Source: CAD feature listing. Evaluate the final solid. Frame: model axes, mm. Face numbers are marked on the shaded views. A direction names the side the tool comes from. Round coordinates to 2 decimals unless told otherwise and drop trailing zeros. Write each loop counter-clockwise with the first axis right and the second up, starting at its lowest first coordinate (ties: lowest second). Pieces come first, ordered by that corner, then holes.
from build123d import *

# Parameters (mm, degrees)
ESQUISSE1_W                     = 500
ESQUISSE1_H                     = 240
EXTRUSION1_DEPTH                = 2
ESQUISSE2_R                     = 36
EXTRUSION2_DEPTH                = 2
ESQUISSE3_R                     = 5
ENL_V_MAT_EXTRU_1_DEPTH         = 2
EXTRUSION3_DEPTH                = 500
CONG_1_R                        = 2
ESQUISSE5_R                     = 3.25
ENL_V_MAT_EXTRU_2_DEPTH         = 2
ENL_V_MAT_EXTRU_3_DEPTH         = 2
R_P_TITION_LIN_AIRE1_COUNT      = 2
R_P_TITION_LIN_AIRE1_PITCH      = 101
R_P_TITION_LIN_AIRE1_COUNT_DIR2 = 2
R_P_TITION_LIN_AIRE1_PITCH_DIR2 = 55
ENL_V_MAT_EXTRU_4_DEPTH         = 2
R_P_TITION_LIN_AIRE2_COUNT      = 2
R_P_TITION_LIN_AIRE2_PITCH      = 55
R_P_TITION_LIN_AIRE2_COUNT_DIR2 = 2
R_P_TITION_LIN_AIRE2_PITCH_DIR2 = 101
ESQUISSE8_R                     = 2.75
ENL_V_MAT_EXTRU_5_DEPTH         = 2
ESQUISSE9_R                     = 2.75
ENL_V_MAT_EXTRU_6_DEPTH         = 2
ESQUISSE10_R                    = 1.6
ENL_V_MAT_EXTRU_7_DEPTH         = 394.248331319
ESQUISSE11_R                    = 2.25
ENL_V_MAT_EXTRU_8_DEPTH         = 10


with BuildPart() as part:
    # Esquisse1 → Extrusion1 (new body)
    with BuildSketch(Plane.XY):
        Rectangle(ESQUISSE1_W, ESQUISSE1_H)
    extrude(amount=EXTRUSION1_DEPTH)

    # Esquisse2 → Extrusion2 (add)
    with BuildSketch(Plane.ZY.offset(250)):
        with BuildLine():
            Line((122, -152.166849215), (122, -175.698605572))
            ThreePointArc((122, -175.698605572), (55.48059391, -159.938789336), (0, -120))
            Line((0, -120), (0, 120))
            ThreePointArc((0, 120), (55.48059391, 159.938789336), (122, 175.698605572))
            Line((122, 175.698605572), (122, 152.166849215))
            ThreePointArc((122, 152.166849215), (247.5, 0), (122, -152.166849215))
        make_face()
        with Locations(Location((92.5, 0, 0), (0, 0, 270))):
            Circle(ESQUISSE2_R, mode=Mode.SUBTRACT)
    extrusion2 = extrude(amount=EXTRUSION2_DEPTH)

    # Esquisse3 → Enlèv. mat.-Extru.1 (cut)
    with BuildSketch(Plane.ZY.offset(252)):
        with Locations(Location((110, 140, 0), (0, 0, 270))):
            Circle(ESQUISSE3_R)
        with Locations(Location((110, -140, 0), (0, 0, 90))):
            Circle(ESQUISSE3_R)
    enl_v_mat_extru_1 = extrude(amount=-ENL_V_MAT_EXTRU_1_DEPTH, mode=Mode.SUBTRACT)

    # Symétrie1: Extrusion2, Enlèv. mat.-Extru.1 across plane
    add(extrusion2.mirror(Plane(origin=(0, 0, 0), x_dir=(0, 0, 1), z_dir=(1, 0, 0))))
    add(enl_v_mat_extru_1.mirror(Plane(origin=(0, 0, 0), x_dir=(0, 0, 1), z_dir=(1, 0, 0))), mode=Mode.SUBTRACT)

    # Esquisse4 → Extrusion3 (add)
    with BuildSketch(Plane(origin=(-250, 0, 0), x_dir=(0, 0, -1), z_dir=(1, 0, 0))):
        Polygon((-2, -120), (-67.268218737, -139.080346508), (-66.707032075, -141), (0, -121.499034429), (0, -120), align=None)
    extrusion3 = extrude(amount=EXTRUSION3_DEPTH)

    # Symétrie2: Extrusion3 across plane
    add(extrusion3.mirror(Plane.ZX))

    # Congé1
    cong_1_edges = [part.edges().sort_by_distance(p)[0] for p in [
        (-252, 0, 0),
        (252, 0, 0),
        (0, -121.499034429, 0),
        (0, 121.499034429, 0),
    ]]
    fillet(cong_1_edges, radius=CONG_1_R)

    # Esquisse5 → Enlèv. mat.-Extru.2 (cut)
    with BuildSketch(Plane.XY.offset(2)):
        with Locations((-48, 28)):
            Circle(ESQUISSE5_R)
        with Locations(Location((48, 28, 0), (0, 0, 180))):
            Circle(ESQUISSE5_R)
        with Locations((48, -28)):
            Circle(ESQUISSE5_R)
        with Locations(Location((-48, -28, 0), (0, 0, 180))):
            Circle(ESQUISSE5_R)
    extrude(amount=-ENL_V_MAT_EXTRU_2_DEPTH, mode=Mode.SUBTRACT)

    # Esquisse6 → Enlèv. mat.-Extru.3 (cut)
    with BuildSketch(Plane.XY.offset(2)):
        with BuildLine():
            Line((189, 85), (196, 85))
            ThreePointArc((196, 85), (200, 81), (196, 77))
            Line((196, 77), (189, 77))
            ThreePointArc((189, 77), (185, 81), (189, 85))
        make_face()
    enl_v_mat_extru_3 = extrude(amount=-ENL_V_MAT_EXTRU_3_DEPTH, mode=Mode.SUBTRACT)

    # Répétition linéaire1: Enl_v. mat.-Extru.3 2 × 2
    with Locations(*[(-j * R_P_TITION_LIN_AIRE1_PITCH_DIR2, -i * R_P_TITION_LIN_AIRE1_PITCH, 0) for i in range(R_P_TITION_LIN_AIRE1_COUNT) for j in range(R_P_TITION_LIN_AIRE1_COUNT_DIR2) if (i, j) != (0, 0)]):
        add(enl_v_mat_extru_3, mode=Mode.SUBTRACT)

    # Esquisse7 → Enlèv. mat.-Extru.4 (cut)
    with BuildSketch(Plane.XY.offset(2)):
        with BuildLine():
            Line((-196, -77), (-189, -77))
            ThreePointArc((-189, -77), (-185, -81), (-189, -85))
            Line((-189, -85), (-196, -85))
            ThreePointArc((-196, -85), (-200, -81), (-196, -77))
        make_face()
    enl_v_mat_extru_4 = extrude(amount=-ENL_V_MAT_EXTRU_4_DEPTH, mode=Mode.SUBTRACT)

    # Répétition linéaire2: Enl_v. mat.-Extru.4 2 × 2
    with Locations(*[(i * R_P_TITION_LIN_AIRE2_PITCH, j * R_P_TITION_LIN_AIRE2_PITCH_DIR2, 0) for i in range(R_P_TITION_LIN_AIRE2_COUNT) for j in range(R_P_TITION_LIN_AIRE2_COUNT_DIR2) if (i, j) != (0, 0)]):
        add(enl_v_mat_extru_4, mode=Mode.SUBTRACT)

    # Esquisse8 → Enlèv. mat.-Extru.5 (cut)
    with BuildSketch(Plane.XY.offset(2)):
        with Locations((-241, 87.5)):
            Circle(ESQUISSE8_R)
        with Locations((-71, 87.5)):
            Circle(ESQUISSE8_R)
    extrude(amount=-ENL_V_MAT_EXTRU_5_DEPTH, mode=Mode.SUBTRACT)

    # Esquisse9 → Enlèv. mat.-Extru.6 (cut)
    with BuildSketch(Plane.XY.offset(2)):
        with Locations((71, -87.5)):
            Circle(ESQUISSE9_R)
        with Locations((241, -87.5)):
            Circle(ESQUISSE9_R)
    extrude(amount=-ENL_V_MAT_EXTRU_6_DEPTH, mode=Mode.SUBTRACT)

    # Esquisse10 → Enlèv. mat.-Extru.7 (cut, through all)
    with BuildSketch(Plane.XY.offset(2)):
        with Locations((-169, 48)):
            Circle(ESQUISSE10_R)
        with Locations((-161, 48)):
            Circle(ESQUISSE10_R)
        with Locations((161, -48)):
            Circle(ESQUISSE10_R)
        with Locations((169, -48)):
            Circle(ESQUISSE10_R)
    extrude(amount=-ENL_V_MAT_EXTRU_7_DEPTH, mode=Mode.SUBTRACT)

    # Esquisse11 → Enlèv. mat.-Extru.8 (cut)
    with BuildSketch(Plane.XY.offset(2)):
        with Locations((0, -75)):
            Circle(ESQUISSE11_R)
        with Locations((0, -85)):
            Circle(ESQUISSE11_R)
    extrude(amount=-ENL_V_MAT_EXTRU_8_DEPTH, mode=Mode.SUBTRACT)


solid = part.part
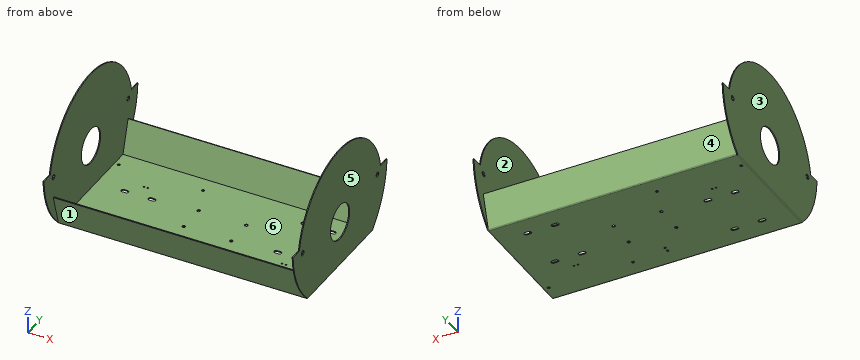
1) Material intervals for line 1 (X direction, y = 73, z = 51); line 2 (Z direction, x = 69, y = -41); line 3 (Y direction, x = 220.5, z = 39.5), sorted ascending.
Taken from the geometry:
line 1: x = -252 to -250, 250 to 252
line 2: z = 0 to 2
line 3: y = -133.05 to -130.96, 130.96 to 133.05
2) Pull-direction query (Y, two-part tool) for the marked faces 1, 2 and 3; classes: released by +Y, released by -Y, zero draft, split by the parting line, or undercut.
Taken from the geometry:
face 1: released by -Y
face 2: undercut
face 3: zero draft
3) Section query D-D on y = -60. Return the cut outline in (x, z).
Taken from the geometry:
outline: (-252, 2) arc R2 ccw to (-250, 0) - (250, 0) arc R2 ccw to (252, 2) - (252, 235.42) - (250, 235.42) - (250, 2) - (-250, 2) - (-250, 235.42) - (-252, 235.42) - close
4) Section query C-C on x = -118. Return the cut outline in (y, z).
Taken from the geometry:
outline: (-141, 66.71) - (-121.92, 1.44) arc R2 ccw to (-120, 0) - (120, 0) arc R2 ccw to (121.92, 1.44) - (141, 66.71) - (139.08, 67.27) - (120, 2) - (-120, 2) - (-139.08, 67.27) - close
5) Contact query for flat-ended pins moving along their axis: P1, Ø1.6, axis at x = 136.5, z = 1.5, coming from the +Y side; P2, Ø1, axis at x = -193, z = 1.5, coming from the +Y side; P3, Ø4.5, axis at x = 241, y = -87.5, coming from the -Z side; P4, Ø0.6, axis at x = 138, z = 1.5, coming from the -Y side. Output: stop coordinate, or through.
Taken from the geometry:
P1: stops at y = 122.17
P2: stops at y = 122.08
P3: passes through
P4: stops at y = -122.03
6) Section query B-B on z = 213. Return the cut outline in (x, y).
Taken from the geometry:
outline: (-252, -97.49) - (-250, -97.49) - (-250, 97.49) - (-252, 97.49) - close; (250, -97.49) - (252, -97.49) - (252, 97.49) - (250, 97.49) - close
7) Section query A-A on y = 0. Return the cut outline in (x, z).
Taken from the geometry:
outline: (-252, 2) arc R2 ccw to (-250, 0) - (250, 0) arc R2 ccw to (252, 2) - (252, 56.5) - (250, 56.5) - (250, 2) - (-250, 2) - (-250, 56.5) - (-252, 56.5) - close; (-252, 128.5) - (-250, 128.5) - (-250, 247.5) - (-252, 247.5) - close; (250, 128.5) - (252, 128.5) - (252, 247.5) - (250, 247.5) - close
8) Reachability of the marked faces 4, 5 and 6 from +Z, -Z, +X, -X, +Y, -Y: full face, straight path, thin tool, end or side. Return the list, or none.
Taken from the geometry:
face 4: -Z, +Y
face 5: +Z, -Z, +X, +Y, -Y
face 6: +Z
